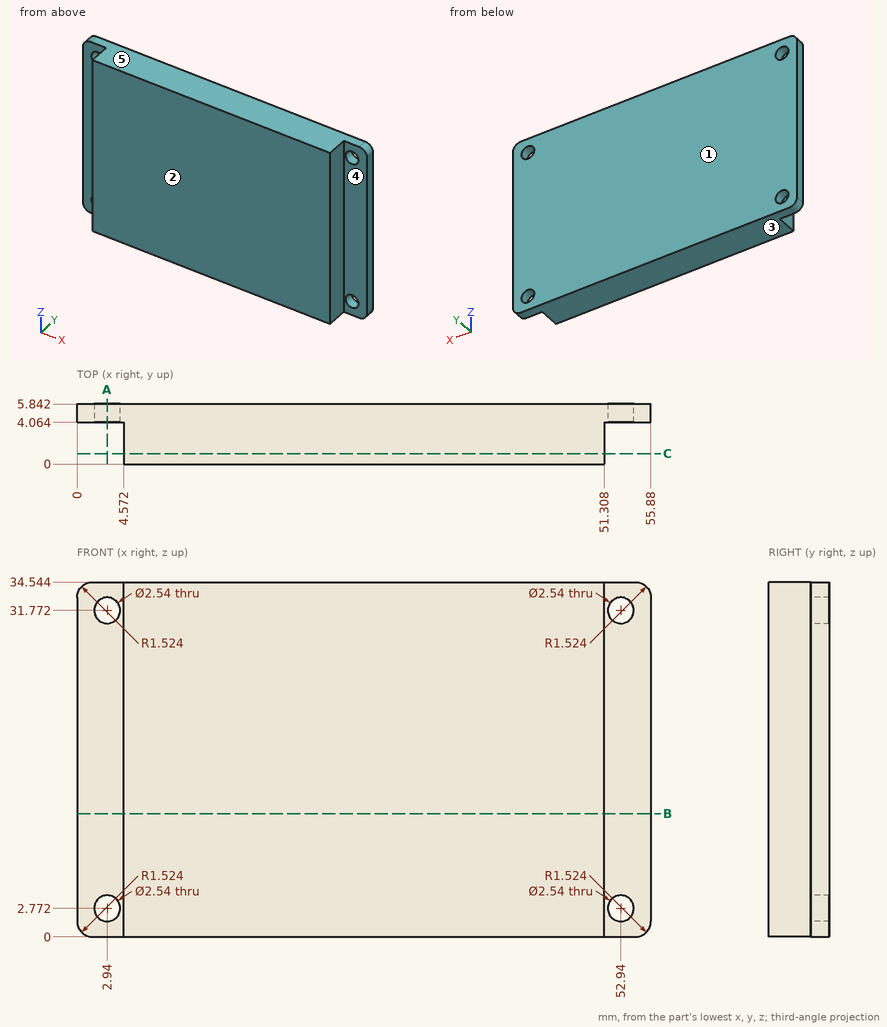
The figure shows three views and two pictorial views of one solid part (mm, origin at its lowest corner). Answer the questions. A direction names the side the tool comes from. Round coordinates to 2 decimals unless told otherwise and drop trailing zeros. Order: outer loops, then holes, each group sorted by start corner. A loop starts at its lowest first (then second) coordinate and runs counter-clockwise, first axis right, second up.
Q1. The mould has two halves that part along Y. Classify the marked faces 1, 2 and 3: pulls with the +Y half, pulls with the -Y half, needs draft (parallel to the pull), parting line crosses it, or undercut.
Solution:
face 1: pulls with the +Y half
face 2: pulls with the -Y half
face 3: needs draft
Q2. A cutting plane is placed at C-C, the plane y = 1. Determine the outline of the cut face in (x, z), then the cut area to 3 significant figures.
Solution:
outline: (4.57, 0) - (51.31, 0) - (51.31, 34.54) - (4.57, 34.54) - close
area: 1,610 mm2
Q3. Find the intervals of material crossed by line 1 along Z through (x, y) = (2.94, 4.6); line 2 along X through (y, z) = (3.9, 14); line 3 along Y through (x, z) = (53, 7), in increasing order.
Solution:
line 1: z = 0 to 1.5, 4.04 to 30.5, 33.04 to 34.54
line 2: x = 4.57 to 51.31
line 3: y = 4.06 to 5.84
Q4. A cutting plane is placed at B-B, the plane z = 12. Determine the outline of the cut face in (x, y), then the cut area to 3 significant figures.
Solution:
outline: (0, 4.06) - (4.57, 4.06) - (4.57, 0) - (51.31, 0) - (51.31, 4.06) - (55.88, 4.06) - (55.88, 5.84) - (0, 5.84) - close
area: 289 mm2
Q5. A tool of negligible diameter and unlimited length cuts with its end or side. For the marked faces 4 and 5, from which of +Z, -Z, +X, -X, +Y, -Y can it reach the whole face along a straight path? Write none if from no direction.
Solution:
face 4: +Z, -Z, +X, -Y
face 5: +Z, +X, -X, +Y, -Y
Q6. Given pin 1 Ø2.5 at (x, z) = (2, 16.5) entering from -Y; pin 2 Ø1.2 at (y, z) = (2.5, 11) entering from +X; pin 3 Ø2 at (y, z) = (2.5, 20.5) entering from -X, each flat-ended and moving along its own axis, determine where each tip first touches the part or whether it passes through.
Solution:
pin 1: stops at y = 4.06
pin 2: stops at x = 51.31
pin 3: stops at x = 4.57
Q7. A cutting plane is placed at A-A, the plane x = 2.94. Determine the outline of the cut face in (y, z).
Solution:
outline: (4.06, 0) - (5.84, 0) - (5.84, 1.5) - (4.06, 1.5) - close; (4.06, 4.04) - (5.84, 4.04) - (5.84, 30.5) - (4.06, 30.5) - close; (4.06, 33.04) - (5.84, 33.04) - (5.84, 34.54) - (4.06, 34.54) - close
